Geometry: see drawing. Coordinates: mm, zero at the bounding-box minimum. Give positions to 0.01 mm unless a question says otherwise; leave off trailing zeros. Order: outer loops, then holes, each group sorted by start corner. A loop starts at its lowest first (then second) coordinate and runs counter-clockwise, first axis right, second up. Notation, with made-up numbers: (61.25, 39.5) -> (109.25, 39.5) arc R20 cw to (109.25, 56.5) -> close; hole circle Ø1 at (3.5, 12). An arc over 180 degrees is marked (long way). One line per item, written item: value. Start each with the question number.
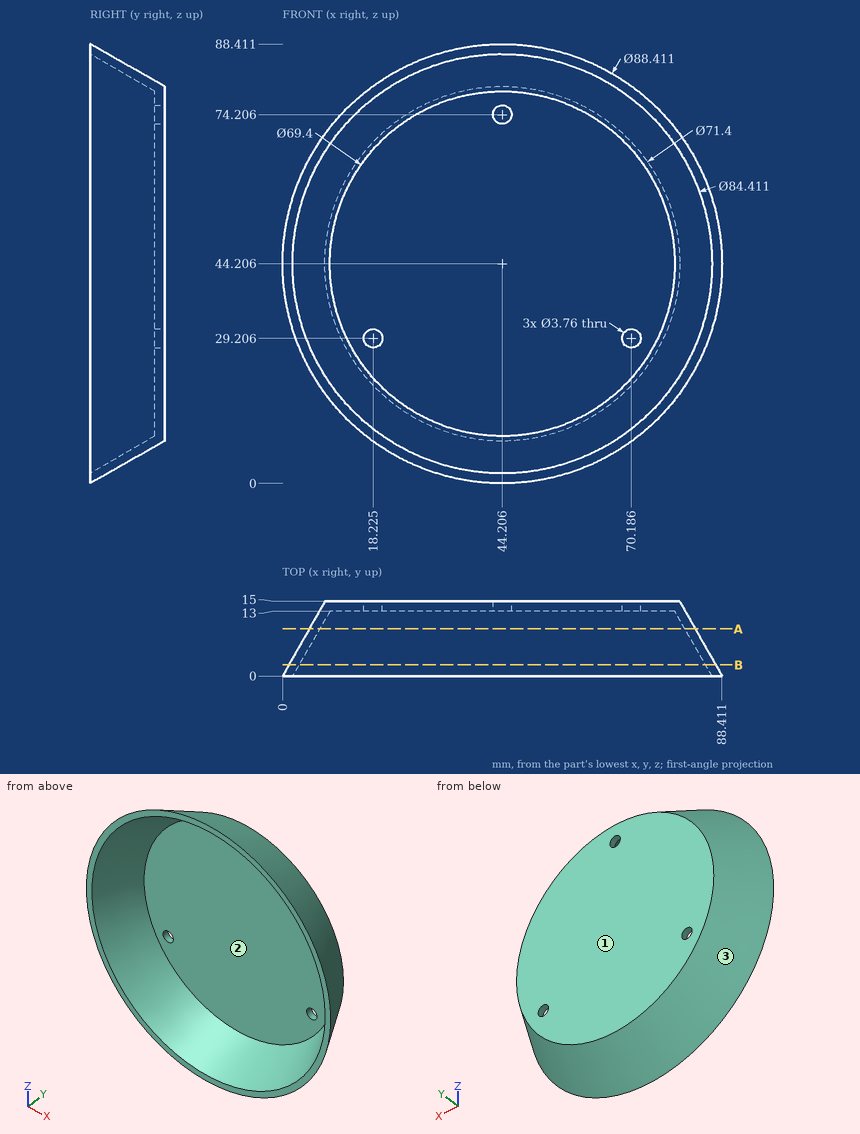
1. Pin query (flat end, axial travel): P1, Ø6, axis at x = 24.5, y = 2, coming from the +Z side; P2, Ø6, axis at y = 7.5, z = 65, coming from the -X side (1 decimal); P3, Ø1, axis at y = 5, z = 29.5, coming from the +X side. Return the tip coordinate at first contact, or that it passes through.
2. Cut plane B-B, the plane y = 2.25. Return loops of the section in (x, z) (1 decimal).
3. Draft query along Z for the marked faces 1, 2 and 3. Return one class per face: pulls with the +Z half, pulls with the -Z half, needs draft (parallel to the pull), parting line crosses it, or undercut.
4. Material intervals for L1, parallel to Y at x = 32, z = 27.5; L2, parallel to X at y = 7.5, z = 26.5 (1 decimal); L3, parallel to X at y = 7.25, z = 24 (1 decimal), sorted ascending. Write a range as [from, to].
5. Cut plane A-A, the plane y = 9.5. Return loops of the section in (x, z) (1 decimal).
Answers follow:
1. P1: stops at z = 84.81
1. P2: stops at x = 7.5
1. P3: stops at x = 83.23
2. outline: circle Ø85.9 at (44.2, 44.2); hole circle Ø81.8 at (44.2, 44.2)
3. face 1: needs draft
3. face 2: undercut
3. face 3: parting line crosses it
4. L1: y = [13, 15]
4. L2: x = [8.4, 10.7], [77.7, 80]
4. L3: x = [9.6, 12], [76.4, 78.8]
5. outline: circle Ø77.6 at (44.2, 44.2); hole circle Ø73.4 at (44.2, 44.2)
